Read the model definition and answer for the solid it produces. Units are mm, in the model's axes. Face numbers are marked on the shaded views. Give positions to 0.01 mm unless a question says otherwise; leave off trailing zeros. Loops run counter-clockwise (first coordinate to the right, second up) from the corner with the lowest first, then second, coordinate; pieces in that order, holes last. Notation, with made-up numbers: (18, 39.5) -> (38, 39.5) arc R9 ccw to (38, 53.5) -> close; hole circle Ø6 at (32.5, 24.5). An arc over 180 degrees is marked (long way). Return JSON: item names as keys, results as strings. Group by question number.
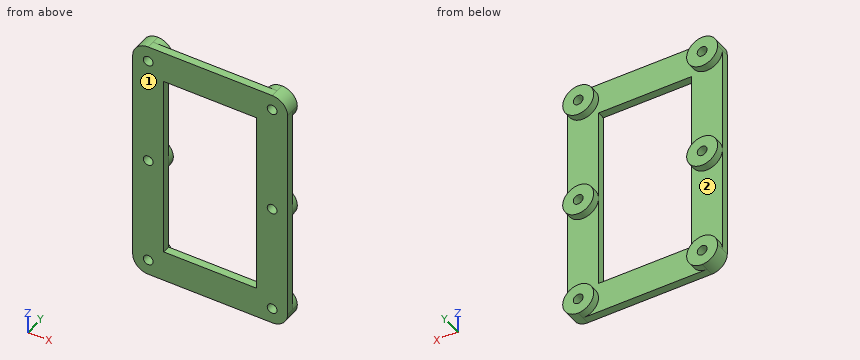
from build123d import *

# Parameters (mm, degrees)
SKETCH1_W              = 63.5
SKETCH1_H              = 101.6
BOSS_EXTRUDE1_DEPTH    = 6.35
FILLET1_R              = 6.35
F_10_32_TAPPED_HOLE1_D = 4.0386
SKETCH10_W             = 38.1
SKETCH10_H             = 76.2
CUT_EXTRUDE1_DEPTH     = 7.35
CUT_EXTRUDE2_DEPTH     = 3.175


with BuildPart() as part:
    # Sketch1 → Boss-Extrude1 (new body)
    with BuildSketch(Plane(origin=(0, 0, 0), x_dir=(1, 0, 0), z_dir=(0, 1, 0))):
        Rectangle(SKETCH1_W, SKETCH1_H)
    extrude(amount=BOSS_EXTRUDE1_DEPTH)

    # Fillet1
    fillet1_edges = [part.edges().sort_by_distance(p)[0] for p in [
        (-31.75, 3.175, -50.8),
        (31.75, 3.175, -50.8),
        (31.75, 3.175, 50.8),
        (-31.75, 3.175, 50.8),
    ]]
    fillet(fillet1_edges, radius=FILLET1_R)

    # #10-32 Tapped Hole1 (through all)
    with Locations(Plane(origin=(0, 6.35, 0), x_dir=(1, 0, 0), z_dir=(0, 1, 0))):
        with Locations((25.4, 44.45), (-25.4, 44.45), (-25.4, -44.45), (25.4, -44.45), (-25.4, 0), (25.4, 0)):
            Hole(F_10_32_TAPPED_HOLE1_D / 2)

    # Sketch10 → Cut-Extrude1 (cut, through all)
    with BuildSketch(Plane(origin=(0, 6.35, 0), x_dir=(1, 0, 0), z_dir=(0, 1, 0))):
        Rectangle(SKETCH10_W, SKETCH10_H)
    extrude(amount=-CUT_EXTRUDE1_DEPTH, mode=Mode.SUBTRACT)

    # Sketch11 → Cut-Extrude2 (cut)
    with BuildSketch(Plane(origin=(0, 6.35, 0), x_dir=(1, 0, 0), z_dir=(0, 1, 0))):
        with BuildLine():
            ThreePointArc((25.4, -50.8), (20.909871939, -39.959871939), (31.75, -44.45))
            Line((31.75, -44.45), (31.75, 0))
            ThreePointArc((31.75, 0), (25.4, -6.35), (19.05, 0))
            Line((19.05, 0), (19.05, -38.1))
            Line((19.05, -38.1), (-19.05, -38.1))
            Line((-19.05, -38.1), (-19.05, 0))
            ThreePointArc((-19.05, 0), (-25.4, -6.35), (-31.75, 0))
            Line((-31.75, 0), (-31.75, -44.45))
            ThreePointArc((-31.75, -44.45), (-20.909871939, -39.959871939), (-25.4, -50.8))
            Line((-25.4, -50.8), (25.4, -50.8))
        make_face()
        with BuildLine():
            ThreePointArc((19.05, 0), (25.4, 6.35), (31.75, 0))
            Line((31.75, 0), (31.75, 44.45))
            ThreePointArc((31.75, 44.45), (20.909871939, 39.959871939), (25.4, 50.8))
            Line((25.4, 50.8), (-25.4, 50.8))
            ThreePointArc((-25.4, 50.8), (-20.909871939, 39.959871939), (-31.75, 44.45))
            Line((-31.75, 44.45), (-31.75, 0))
            ThreePointArc((-31.75, 0), (-25.4, 6.35), (-19.05, 0))
            Line((-19.05, 0), (-19.05, 38.1))
            Line((-19.05, 38.1), (19.05, 38.1))
            Line((19.05, 38.1), (19.05, 0))
        make_face()
    extrude(amount=-CUT_EXTRUDE2_DEPTH, mode=Mode.SUBTRACT)


solid = part.part
1. Flat-ended cylindrical pins translate along their axes: pin 1 Ø3 at (x, z) = (25.4, 0) entering from +Y; pin 2 Ø3 at (x, z) = (0, -37) entering from +Y (3 decimals); pin 3 Ø1 at (y, z) = (5.5, 40) entering from -X. Find the tip coordinate at first contact, or state that the pin passes through.
2. Straight lines are drawn through the part: line 1 (Z direction, x = -25.4, y = 4.25); line 2 (Z direction, x = -25.5, y = 0.5); line 3 (X direction, y = 2.25, z = 44.45). For each, find the intervals that lie inside material, in ascending order. Write a range as from..to.
3. Section C-C on z = 19.5 is taken. Determine the outline of the cut face in (x, y) (3 decimals).
4. Determine the mould class of the marked faces 1 and 2 for opening direction Z: pulls with the +Z half, pulls with the -Z half, needs draft (parallel to the pull), parting line crosses it, or undercut.
5. Section A-A on y = 5.25 is taken. State how many separate pieces and enclosed holes the cut face has, then the cut area to 3 significant figures.
6. Section B-B on x = -9 is taken. Determine the outline of the cut face in (y, z) (3 decimals).
Completed:
{
 "1": {"pin 1": "passes through", "pin 2": "stops at y = 3.175", "pin 3": "stops at x = -30.37"},
 "2": {"line 1": "z = -50.8..-46.47, -42.43..-38.1, -6.35..-2.02, 2.02..6.35, 38.1..42.43, 46.47..50.8", "line 2": "z = -50.8..-46.47, -42.43..-2.02, 2.02..42.43, 46.47..50.8", "line 3": "x = -31.75..-27.42, -23.38..23.38, 27.42..31.75"},
 "3": {"outline": "(-31.75, 0) -> (-19.05, 0) -> (-19.05, 3.175) -> (-31.75, 3.175) -> close; (19.05, 0) -> (31.75, 0) -> (31.75, 3.175) -> (19.05, 3.175) -> close"},
 "4": {"face 1": "needs draft", "face 2": "undercut"},
 "5": {"separate pieces": "6", "enclosed holes": "6", "area": "683 mm²"},
 "6": {"outline": "(0, -50.8) -> (3.175, -50.8) -> (3.175, -38.1) -> (0, -38.1) -> close; (0, 38.1) -> (3.175, 38.1) -> (3.175, 50.8) -> (0, 50.8) -> close"}
}
